Could you check a few things on this model? Use its own coordinates, in mm. Face numbers are marked on the shaded views. A direction names the side the tool comes from. Round coordinates to 2 decimals unless told otherwise and drop trailing zeros. Order: outer loops, then holes, each group sorted by start corner. A loop starts at its lowest first (then second) coordinate and runs counter-clockwise, first axis right, second up. Notation, with made-up numbers: (-32.5, 26) -> (22.5, 26) arc R19 cw to (22.5, 30) -> close; hole circle Ø1 at (-10, -17). An arc over 180 degrees is marked (long way). Put each result on its own line as item: value. Start each with the question number.
from build123d import *

# Parameters (mm, degrees)
SKETCH1_R           = 1.75
BOSS_EXTRUDE1_DEPTH = 10


with BuildPart() as part:
    # Sketch1 → Boss-Extrude1 (new body)
    with BuildSketch(Plane.XY):
        with BuildLine():
            Line((92.526484321, 102.652653788), (111.526484321, 102.652653788))
            ThreePointArc((111.526484321, 102.652653788), (113.647804665, 101.773974132), (114.526484321, 99.652653788))
            Line((114.526484321, 99.652653788), (114.526484321, 90.652653788))
            ThreePointArc((114.526484321, 90.652653788), (113.647804665, 88.531333445), (111.526484321, 87.652653788))
            Line((111.526484321, 87.652653788), (104.655721469, 87.652653788))
            ThreePointArc((104.655721469, 87.652653788), (99.705974001, 85.602401257), (97.655721469, 80.652653788))
            Line((97.655721469, 80.652653788), (97.655721469, 35.652653788))
            ThreePointArc((97.655721469, 35.652653788), (96.777041813, 33.531333445), (94.655721469, 32.652653788))
            Line((94.655721469, 32.652653788), (91.883588365, 32.652653788))
            ThreePointArc((91.883588365, 32.652653788), (91.176481584, 32.945547007), (90.883588365, 33.652653788))
            Line((90.883588365, 33.652653788), (90.883588365, 37.44429483))
            ThreePointArc((90.883588365, 37.44429483), (90.904227909, 37.646416321), (90.96529456, 37.840194422))
            ThreePointArc((90.96529456, 37.840194422), (93.100756161, 50.01744431), (89.526484321, 61.852569654))
            Line((89.526484321, 61.852569654), (89.526484321, 99.652653788))
            ThreePointArc((89.526484321, 99.652653788), (90.405163978, 101.773974132), (92.526484321, 102.652653788))
        make_face()
        with Locations((94.655721469, 97.131560256)):
            Circle(SKETCH1_R, mode=Mode.SUBTRACT)
        with Locations((109.087030876, 94.921659672)):
            Circle(SKETCH1_R, mode=Mode.SUBTRACT)
    extrude(amount=BOSS_EXTRUDE1_DEPTH)


solid = part.part
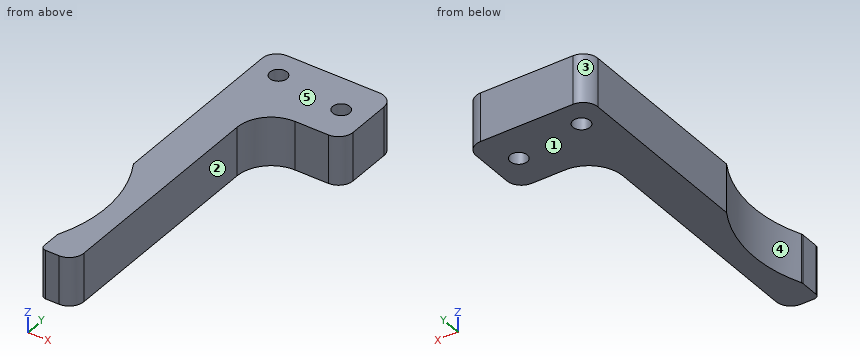
1. Thinking about a two-plate mould opening in Y: for the marked faces 3, 4 and 5, which applies, +Y half, -Y half, draft (parallel to the pull), parting line (faces both ways), or undercut?
2. Which directions (+Z, -Z, +X, -X, +Y, -Y) give clear straight access to the entire face, cutting with the end or side of a thin tool? Please do the marked faces 1 and 2.
3. For pin 1 Ø1.5 at (y, z) = (85.5, 4.5) entering from +X; pin 2 Ø3 at (x, y) = (94.66, 97.13) entering from -Z; pin 3 Ø2 at (x, z) = (109, 4.5) entering from -Y; pin 4 Ø1.1 at (y, z) = (36, 7.5) entering from -X, each with a flat end and sliding along its axis, tell me the tip position at first contact or that it passes through.
4. I need wall thicknesses on L1, parallel to X at y = 95, z = 1.75; L2, parallel to X at y = 79.5, z = 3; L3, parallel to X at y = 94.5, z = 7.75. Which ranges of each line are inside material? Lowest first, please.
5. If we section it at C-C, the plane x = 101.75: Please give me the cut outline in (y, z), then the cut area to 3 significant figures.
6. If we section it at A-A, the plane z = 2: Please give me the cut outline in (x, y).
7. If we section it at B-B, the plane y = 65: Please give me the cut outline in (x, z).
Results below:
1. face 3: +Y half
1. face 4: undercut
1. face 5: draft
2. face 1: -Z, +X, -X, +Y, -Y
2. face 2: +Z, -Z, +X, -Y
3. pin 1: x = 100.45
3. pin 2: through
3. pin 3: y = 87.65
3. pin 4: x = 90.88
4. L1: 89.53 to 107.34, 110.84 to 114.53
4. L2: 89.53 to 97.66
4. L3: 89.53 to 107.39, 110.79 to 114.53
5. outline: (87.02, 0) -> (102.65, 0) -> (102.65, 10) -> (87.02, 10) -> close
5. area: 156 mm2
6. outline: (89.53, 61.85) arc R26.72 cw to (90.97, 37.84) arc R1 ccw to (90.88, 37.44) -> (90.88, 33.65) arc R1 ccw to (91.88, 32.65) -> (94.66, 32.65) arc R3 ccw to (97.66, 35.65) -> (97.66, 80.65) arc R7 cw to (104.66, 87.65) -> (111.53, 87.65) arc R3 ccw to (114.53, 90.65) -> (114.53, 99.65) arc R3 ccw to (111.53, 102.65) -> (92.53, 102.65) arc R3 ccw to (89.53, 99.65) -> close; hole circle Ø3.5 at (94.66, 97.13); hole circle Ø3.5 at (109.09, 94.92)
7. outline: (89.53, 0) -> (97.66, 0) -> (97.66, 10) -> (89.53, 10) -> close
